Design review of the part built by this model. Coordinates are the model's own, in mm. Face numbers are marked on the shaded views. A direction names the side the tool comes from. Round coordinates to 2 decimals unless told otherwise and drop trailing zeros. Loops run counter-clockwise (first coordinate to the right, second up) from the corner with the lowest first, then second, coordinate; pieces in that order, holes last. Notation, with made-up numbers: (-8.5, 86.25) - (5.5, 86.25) arc R14 cw to (5.5, 91.25) - close; hole circle Ø4 at (26.5, 0.5). An arc over 180 degrees is marked (long way). Use one line per item in the form item = value. Start each with the question number.
(1) The part is to be moulded in two halves that separate along X. For the marked faces 1, 2, 3 and 4, say which applies: released by +X, released by -X, zero draft, split by the parting line, or undercut.
(2) We need section B-B, the plane z = -4.5. Write out the cut boundary in (x, y), then the cut area to 3 significant figures.
(3) Machinability: for the marked faces 5, 6 and 7, which of the approach directions +Z, -Z, +X, -X, +Y, -Y give a long, thin tool a straight path to every point of the face, cutting with its end or side? Answer none if there is none.
(4) We need section D-D, the plane x = -19.05. Write out the cut boundary in (y, z).
(5) We need section A-A, the plane x = 0. Write out the cut boundary in (y, z) (3 decimals).
(6) Wall thickness on probe 1 along X at (y, z) = (19, -6); probe 2 along Z at (x, y) = (0, 5) (3 decimals): over which ranges is each line inside the solid? List them lowest first. Write a range as [from, to].
(7) For pin 1 (1.2 mm diameter, centred on x = 19.5, y = 19, fed in from +Z); pin 2 (3.5 mm diameter, centred on x = 19.05, y = 19.05, fed in from -Z); pin 3 (1.5 mm diameter, centred on y = -18.5, z = -26.5, fed in from +X); pin 4 (5 mm diameter, centred on x = 19.05, y = -19.05, fed in from +Z), all flat-tipped, find the tip position at first contact; note any pin that passes through.
(8) We need section C-C, the plane y = -3. Write out the cut boundary in (x, z) (3 decimals), then the cut area to 3 significant figures.
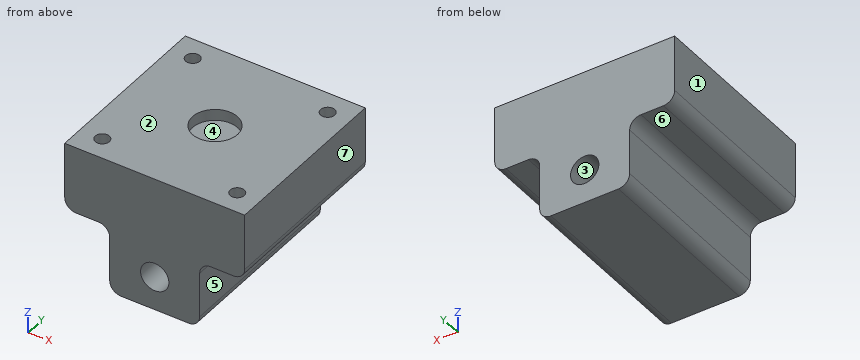
from build123d import *

# Parameters (mm, degrees)
F0_R     = 4
F1_DEPTH = 25.4
F2_R     = 2
F3_DEPTH = 12.7
F4_R     = 6.35
F5_DEPTH = 3.175


with BuildPart() as f1:
    # F0 (on Front) → F1 (new body, symmetric)
    with BuildSketch(Plane.XZ):
        with BuildLine():
            Line((25.4, 0), (-25.4, 0))
            Line((-25.4, 0), (-25.4, -15.875))
            ThreePointArc((-25.4, -15.875), (-24.470064, -18.120064), (-22.225, -19.05))
            Line((-22.225, -19.05), (-15.875, -19.05))
            ThreePointArc((-15.875, -19.05), (-13.629936, -19.979936), (-12.7, -22.225))
            Line((-12.7, -22.225), (-12.7, -34.925))
            ThreePointArc((-12.7, -34.925), (-11.770064, -37.170064), (-9.525, -38.1))
            Line((-9.525, -38.1), (9.525, -38.1))
            ThreePointArc((9.525, -38.1), (11.770064, -37.170064), (12.7, -34.925))
            Line((12.7, -34.925), (12.7, -22.225))
            ThreePointArc((12.7, -22.225), (13.629936, -19.979936), (15.875, -19.05))
            Line((15.875, -19.05), (22.225, -19.05))
            ThreePointArc((22.225, -19.05), (24.470064, -18.120064), (25.4, -15.875))
            Line((25.4, -15.875), (25.4, 0))
        make_face()
        with Locations((0, -28.575)):
            Circle(F0_R, mode=Mode.SUBTRACT)
    extrude(amount=F1_DEPTH, both=True)

    # F2 (on face) → F3 (cut)
    with BuildSketch(Plane.XY):
        with Locations((-19.05, -19.05)):
            Circle(F2_R)
        with Locations((19.05, -19.05)):
            Circle(F2_R)
        with Locations((19.05, 19.05)):
            Circle(F2_R)
        with Locations((-19.05, 19.05)):
            Circle(F2_R)
    extrude(amount=-F3_DEPTH, mode=Mode.SUBTRACT)

    # F4 (on face) → F5 (cut)
    with BuildSketch(Plane.XY):
        Circle(F4_R)
    extrude(amount=-F5_DEPTH, mode=Mode.SUBTRACT)


solid = f1.part
Data:
q1.face_1 = released by -X
q1.face_2 = zero draft
q1.face_3 = undercut
q1.face_4 = undercut
q2.outline = (-25.4, -25.4) - (25.4, -25.4) - (25.4, 25.4) - (-25.4, 25.4) - close; hole circle Ø4 at (-19.05, -19.05); hole circle Ø4 at (-19.05, 19.05); hole circle Ø4 at (19.05, -19.05); hole circle Ø4 at (19.05, 19.05)
q2.area = 2,530 mm^2
q3.face_5 = -Z, +X, +Y, -Y
q3.face_6 = -Z, -X, +Y, -Y
q3.face_7 = +Z, -Z, +X, +Y, -Y
q4.outline = (-25.4, -19.05) - (25.4, -19.05) - (25.4, 0) - (21.05, 0) - (21.05, -12.7) - (17.05, -12.7) - (17.05, 0) - (-17.05, 0) - (-17.05, -12.7) - (-21.05, -12.7) - (-21.05, 0) - (-25.4, 0) - close
q5.outline = (-25.4, -38.1) - (25.4, -38.1) - (25.4, -32.575) - (-25.4, -32.575) - close; (-25.4, -24.575) - (25.4, -24.575) - (25.4, 0) - (6.35, 0) - (6.35, -3.175) - (-6.35, -3.175) - (-6.35, 0) - (-25.4, 0) - close
q6.probe_1 = [-25.4, -21.05], [-17.05, 17.05], [21.05, 25.4]
q6.probe_2 = [-38.1, -32.575], [-24.575, -3.175]
q7.pin_1 = -12.7
q7.pin_2 = -19.05
q7.pin_3 = 12.7
q7.pin_4 = 0
q8.outline = (-25.4, -15.875) arc R3.175 ccw to (-22.225, -19.05) - (-15.875, -19.05) arc R3.175 cw to (-12.7, -22.225) - (-12.7, -34.925) arc R3.175 ccw to (-9.525, -38.1) - (9.525, -38.1) arc R3.175 ccw to (12.7, -34.925) - (12.7, -22.225) arc R3.175 cw to (15.875, -19.05) - (22.225, -19.05) arc R3.175 ccw to (25.4, -15.875) - (25.4, 0) - (5.597, 0) - (5.597, -3.175) - (-5.597, -3.175) - (-5.597, 0) - (-25.4, 0) - close; hole circle Ø8 at (0, -28.575)
q8.area = 1,360 mm^2
